Part model, mm, in its own coordinate system. Round coordinates to 2 decimals unless told otherwise and drop trailing zeros. Write each loop counter-clockwise with the first axis right and the second up, starting at its lowest first coordinate (ties: lowest second). Pieces come first, ordered by that corner, then holes. Notation, with made-up numbers: M 77,75 L 131,75 A22 cw 131,81 Z; hole C 35.25,69 d9. An arc over 180 degrees is marked long. Answer as a JSON object with one key per item and string values. Group by question number.
1. Band-saw the part on B-B, the plane x = 2.5. Write the cut outline in (y, z).
2. Drop flat-ended pins along their axis: pin 1 (1.2 mm diameter, centred on x = -39.5, z = 1.5, fed in from -Y); pin 2 (1.2 mm diameter, centred on x = -11, z = 0.5, fed in from +Y). Give the stop position or say it passes through.
3. Drill centre lines: line 1 (Y direction, x = -11, z = 1.1); line 2 (Y direction, x = 24.5, z = 0.2); line 3 (X direction, y = -8.5, z = 0.85) (3 decimals). Where is each one in solid material? Low to high. Write a range as from..to.
4. Band-saw the part on A-A, the plane y = 14.5. Write the cut outline in (x, z) (3 decimals).
5. Band-saw the part on C-C, the plane x = -27. Write the cut outline in (y, z), plus the area to 3 significant figures.
6. Band-saw the part on D-D, the plane z = 1.8. Count the separate pieces of the cut face and the enclosed holes in it, plus the area to 3 significant figures.
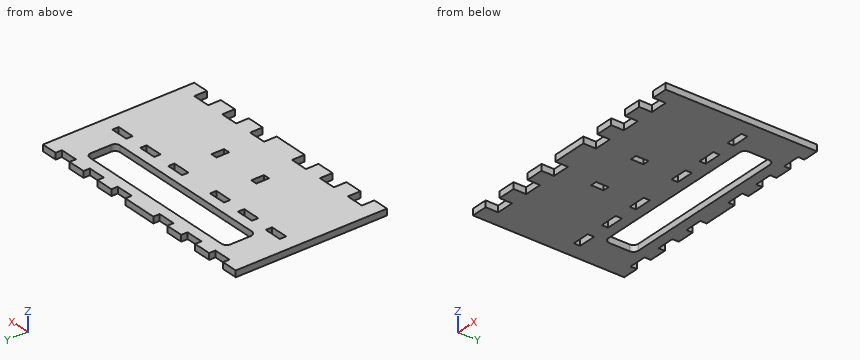
from build123d import *

# Parameters (mm, degrees)
SKETCH1_W           = 7
SKETCH1_H           = 2.5
SKETCH1_W_2         = 2.5
SKETCH1_H_2         = 5
BOSS_EXTRUDE1_DEPTH = 2.5


with BuildPart() as part:
    # Sketch1 → Boss-Extrude1 (new body)
    with BuildSketch(Plane.XY):
        Polygon((-48.325, -30), (-42, -30), (-42, -25), (-35, -25), (-35, -30), (-28, -30), (-28, -25), (-21, -25), (-21, -30), (-14, -30), (-14, -25), (-7, -25), (-7, -30), (7, -30), (7, -25), (14, -25), (14, -30), (21, -30), (21, -25), (28, -25), (28, -30), (35, -30), (35, -25), (42, -25), (42, -30), (48.325, -30), (48.325, 30), (42, 30), (42, 27.5), (35, 27.5), (35, 30), (28, 30), (28, 27.5), (21, 27.5), (21, 30), (14, 30), (14, 27.5), (7, 27.5), (7, 30), (-7, 30), (-7, 27.5), (-14, 27.5), (-14, 30), (-21, 30), (-21, 27.5), (-28, 27.5), (-28, 30), (-35, 30), (-35, 27.5), (-42, 27.5), (-42, 30), (-48.325, 30), align=None)
        with Locations((24.5, 6.25)):
            Rectangle(SKETCH1_W, SKETCH1_H, mode=Mode.SUBTRACT)
        with Locations((38.5, 6.25)):
            Rectangle(SKETCH1_W, SKETCH1_H, mode=Mode.SUBTRACT)
        with Locations((10.5, 6.25)):
            Rectangle(SKETCH1_W, SKETCH1_H, mode=Mode.SUBTRACT)
        with Locations((-38.5, 6.25)):
            Rectangle(SKETCH1_W, SKETCH1_H, mode=Mode.SUBTRACT)
        with Locations((-24.5, 6.25)):
            Rectangle(SKETCH1_W, SKETCH1_H, mode=Mode.SUBTRACT)
        with Locations((-10.5, 6.25)):
            Rectangle(SKETCH1_W, SKETCH1_H, mode=Mode.SUBTRACT)
        with Locations((-10, -10)):
            Rectangle(SKETCH1_W_2, SKETCH1_H_2, mode=Mode.SUBTRACT)
        with BuildLine():
            Line((-33, 11.5), (33, 11.5))
            ThreePointArc((33, 11.5), (34.414213562, 12.085786438), (35, 13.5))
            Line((35, 13.5), (35, 21.5))
            ThreePointArc((35, 21.5), (34.414213562, 22.914213562), (33, 23.5))
            Line((33, 23.5), (-33, 23.5))
            ThreePointArc((-33, 23.5), (-34.414213562, 22.914213562), (-35, 21.5))
            Line((-35, 21.5), (-35, 13.5))
            ThreePointArc((-35, 13.5), (-34.414213562, 12.085786438), (-33, 11.5))
        make_face(mode=Mode.SUBTRACT)
        with Locations((10, -10)):
            Rectangle(SKETCH1_W_2, SKETCH1_H_2, mode=Mode.SUBTRACT)
    extrude(amount=BOSS_EXTRUDE1_DEPTH)


solid = part.part
Worked answers:
{
 "1": {"outline": "M -30,0 L 11.5,0 L 11.5,2.5 L -30,2.5 Z; M 23.5,0 L 30,0 L 30,2.5 L 23.5,2.5 Z"},
 "2": {"pin 1": "stops at y = -25", "pin 2": "stops at y = 27.5"},
 "3": {"line 1": "y = -25..-12.5, -7.5..5, 7.5..11.5, 23.5..27.5", "line 2": "y = -25..5, 7.5..11.5, 23.5..27.5", "line 3": "x = -48.325..-11.25, -8.75..8.75, 11.25..48.325"},
 "4": {"outline": "M -48.325,0 L -35,0 L -35,2.5 L -48.325,2.5 Z; M 35,0 L 48.325,0 L 48.325,2.5 L 35,2.5 Z"},
 "5": {"outline": "M -25,0 L 5,0 L 5,2.5 L -25,2.5 Z; M 7.5,0 L 11.5,0 L 11.5,2.5 L 7.5,2.5 Z; M 23.5,0 L 27.5,0 L 27.5,2.5 L 23.5,2.5 Z", "area": "95.0 mm^2"},
 "6": {"separate pieces": "1", "enclosed holes": "9", "area": "4,520 mm^2"}
}
